Part model, mm, in its own coordinate system. A direction names the side the tool comes from. Coordinates: 2 decimals unless noted, no trailing zeros. Write each loop counter-clockwise with the first axis right and the second up, starting at its lowest first coordinate (ties: lowest second). Pieces come first, ordered by that corner, then holes. Notation, with made-up numbers: M 18,19.5 L 73,19.5 A29 ccw 73,47.5 Z; hole C 87.5,68.5 d10. An arc over 180 degrees is marked long. Use a Markdown table: item, result. Add a question column.
Q1. Slice it at A-A on y = -22. Write the cut outline in (x, z), then the cut area to 3 significant figures.
Q2. Tool access for faces 1 (the cylindrical face through (34.58, -4.394, 1.479)), 2 (the flat face through (1, -12, -13)), 3 (the cylindrical face through (-1.82, -1.48, 80.12)): list every direction of +Z, -Z, +X, -X, +Y, -Y with a clear straight run to the whole face (end or side of a thin tool).
Q3. Mould opens along X. For faces 4 (the cylindrical face through (0.78, 17.48, 88.05)), 5 (the flat face through (-1, 11, -16)), 6 (the flat face through (62.5, -12, -8)) say: released by +X, released by -X, zero draft, split by the parting line, or undercut.
Q4. Wall check: L1, parallel to Y at x = 44.5, z = 1.4; L2, parallel to Z at x = 0, y = -1.1; L3, parallel to Z at x = 0, y = 16.8. Give the ranges that are in metal, low to high. Write a range as from..to.
Q5. Slice it at D-D on y = -12. Write the cut outline in (x, z), then the cut area to 3 significant figures.
Q6. Slice it at C-C on z = 39. Write the cut outline in (x, y).
Q7. Pin check, flat tips, straight feed: pin 1 Ø12.5 at (x, y) = (-50, -15) entering from +Z; pin 2 Ø18.5 at (y, z) = (-21, 47.5) entering from -X; pin 3 Ø15.5 at (x, z) = (0, 94) entering from -Y; pin 4 Ø5 at (x, y) = (44.5, -12.5) entering from +Z. Stop position of each tip, or through.
Q8. Slice it at B-B on x = 0. Write the cut outline in (y, z).
Solid Edge part; units mm, degrees
sketch "Sketch1" plane through (0, 0, 0) normal (1, 0, 0) x (0, 1, 0)
  line L0 (-40, 0) -> (0, 63)
  line L1 (0, 0) -> (0, 63)
  line L2 (-40, 0) -> (0, 0)
extrude "Protrusion1" add sketch "Sketch1" along normal mid plane 12
sketch "Sketch2" plane through (0, 0, 0) normal (1, 0, 0) x (0, 1, 0)
  line L0 (-40, 0) -> (0, 0)
  line L1 (16, 0) -> (0, 0)
  line L2 (16, 0) -> (16, -16)
  line L3 (16, -16) -> (-40, -16)
  line L4 (-40, -16) -> (-40, 0)
extrude "Protrusion_2" add sketch "Sketch2" along normal mid plane 125
sketch "Sketch3" plane through (62.5, -12, 48) normal (1, 0, 0) x (0, 1, 0)
  line L0 (18, -64) -> (18, -61)
  line L1 (18, -61) -> (-18, -61)
  line L2 (-18, -61) -> (-18, -64)
  line L3 (-18, -64) -> (18, -64)
extrude "ExtrudedCutout_1" cut sketch "Sketch3" against normal blind 151
sketch "Sketch4" plane through (0, 0, 56) normal (0, -1, 0) x (1, 0, 0)
  line L0 (-18, 38) -> (-34.25, -56)
  line L1 (30.5, -56) -> (-34.25, -56)
  line L2 (18, 38) -> (30.5, -56)
  arc A0 (-18, 38) -> (18, 38) centre (0, 38) cw
extrude "Protrusion_3" add sketch "Sketch4" against normal blind 16
sketch "Sketch5" plane through (-34.25, -12, 0) normal (0, 0, 1) x (1, 0, 0)
  circle A0 centre (78.75, 0) radius 12.5
  circle A1 centre (78.75, 0) radius 5
  circle A2 centre (-10.25, 0) radius 12.5
  circle A3 centre (-10.25, 0) radius 5
extrude "Protrusion2" add sketch "Sketch5" along normal blind 3
sketch "Sketch6" plane through (-1.875, 0, 56) normal (0, -1, 0) x (1, 0, 0)
  circle A0 centre (1.875, 38) radius 6
  circle A1 centre (1.875, 38) radius 14
extrude "Protrusion_5" add sketch "Sketch6" along normal blind 3
sketch "Sketch7" plane through (0, 16, 48) normal (0, 1, 0) x (-1, 0, 0)
  circle A0 centre (0, 46) radius 6
  circle A1 centre (0, 46) radius 14
extrude "Protrusion3" add sketch "Sketch7" along normal blind 3
fillet "Round_1" radius 5 4 edges at (6, -20, 0) (-6, -20, 0) (30.5, 8, 0) (-34.25, 8, 0)
fillet "Round_2" radius 5 1 edges at (18, 8, 94)
Recorded:
| question | item | result |
|---|---|---|
| 1 | outline | M -62.5,-13 L 62.5,-13 L 62.5,0 L 52,0 L 52,3 L 37,3 L 37,0 L 11,0 A5 cw 6,5 L 6,28.35 L -6,28.35 L -6,5 A5 cw -11,0 L -37,0 L -37,3 L -52,3 L -52,0 L -62.5,0 Z |
| 1 | area | 2,070 mm² |
| 2 | face 1 | +Z |
| 2 | face 2 | -Z, +X, -X |
| 2 | face 3 | -Y |
| 3 | face 4 | undercut |
| 3 | face 5 | zero draft |
| 3 | face 6 | released by +X |
| 4 | L1 | -24.5..-17, -7..0.5 |
| 4 | L2 | -13..61.27, 80..88, 100..108 |
| 4 | L3 | 80..88, 100..108 |
| 5 | outline | M -62.5,-13 L 62.5,-13 L 62.5,0 L 57,0 L 57,3 L 49.5,3 L 49.5,0 L 39.5,0 L 39.5,3 L 32,3 L 32,0 L 11,0 A5 cw 6,5 L 6,44.1 L -6,44.1 L -6,5 A5 cw -11,0 L -32,0 L -32,3 L -39.5,3 L -39.5,0 L -49.5,0 L -49.5,3 L -57,3 L -57,0 L -62.5,0 Z |
| 5 | area | 2,250 mm² |
| 6 | outline | M -27.51,0 L -6,0 L -6,-15.24 L 6,-15.24 L 6,0 L 25.31,0 L 25.31,16 L -27.51,16 Z |
| 7 | pin 1 | z = 3 |
| 7 | pin 2 | through |
| 7 | pin 3 | y = -3 |
| 7 | pin 4 | z = 0 |
| 8 | outline | M -40,-16 L -30,-16 L -30,-13 L 6,-13 L 6,-16 L 16,-16 L 16,80 L 19,80 L 19,88 L 16,88 L 16,100 L 19,100 L 19,108 L 16,108 L 16,112 L 0,112 L 0,108 L -3,108 L -3,100 L 0,100 L 0,88 L -3,88 L -3,80 L 0,80 L 0,63 L -40,0 Z |
